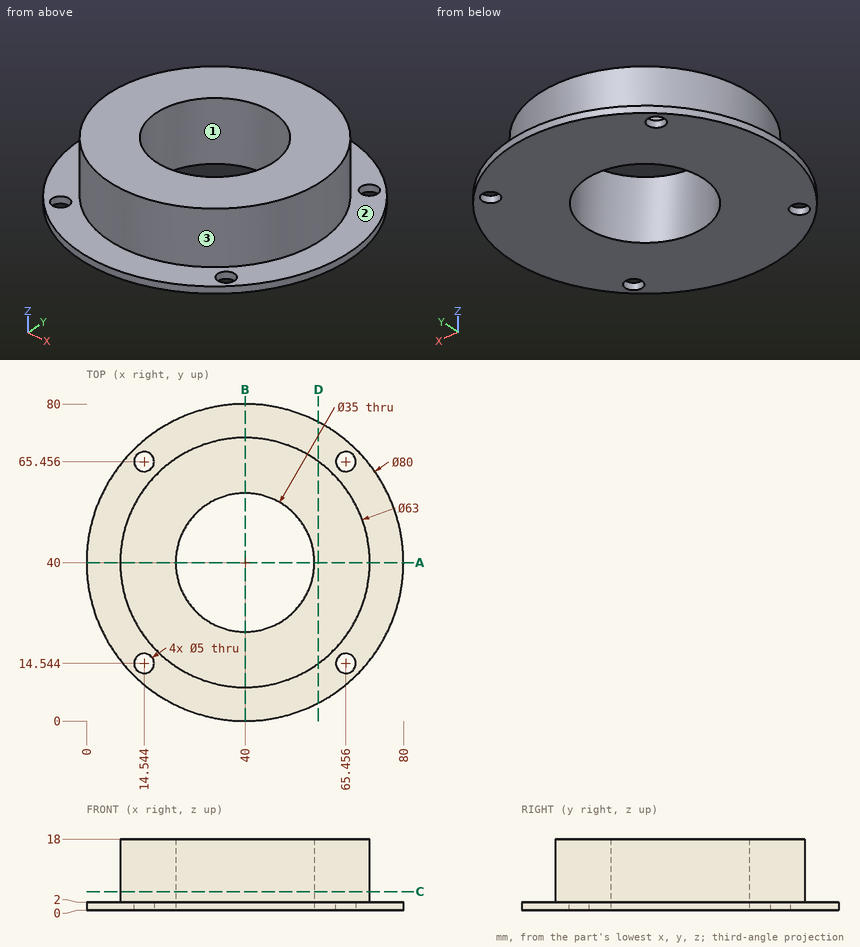
The drawing under review shows one solid part. Ordinate dimensions are in mm from its lowest x, y, z. Coordinates: 2 decimals unless noted, no trailing zeros. Write each loop counter-clockwise with the first axis right and the second up, starting at its lowest first coordinate (ties: lowest second). Pieces come first, ordered by that corner, then holes. Notation, with made-up numbers: (-9, 61) - (7, 61) arc R17 cw to (7, 93) - close; hole circle Ø9 at (34, 47). An arc over 180 degrees is marked (long way). Answer in a Markdown table with one row per item. Add a question column.
Q1. We need section A-A, the plane y = 40. State the section outline as (x, z) points, and give its area (3 significant figures).
Q2. For probe 1 along X at (y, z) = (39.5, 8); probe 2 along Y at (x, z) = (34, 6.75), list the stretches that pass through material, from the lowest coordinate up.
Q3. For P1, Ø3, axis at y = 24.5, z = 5, coming from the -X side; P2, Ø3, axis at y = 66.5, z = 3, coming from the +X side (1 decimal); P3, Ø1, axis at y = 19, z = 7, coming from the +X side, all flat-tipped, find the tip position at first contact; note any pin that passes through.
Q4. We need section D-D, the plane x = 58.5. State the section outline as (y, z) points (1 decimal).
Q5. We need section C-C, the plane z = 4.75. State the section outline as (x, y) points.
Q6. Draft analysis for pull direction Y (two halves, no side actions). For the marked faces 1, 2 and 3, state which applies: +Y half, -Y half, draft (parallel to the pull), parting line (faces both ways), or undercut.
Answer list:
| question | item | result |
|---|---|---|
| 1 | outline | (0, 0) - (22.5, 0) - (22.5, 18) - (8.5, 18) - (8.5, 2) - (0, 2) - close; (57.5, 0) - (80, 0) - (80, 2) - (71.5, 2) - (71.5, 18) - (57.5, 18) - close |
| 1 | area | 538 mm2 |
| 2 | probe 1 | x = 8.5 to 22.51, 57.49 to 71.5 |
| 2 | probe 2 | y = 9.08 to 23.56, 56.44 to 70.92 |
| 3 | P1 | stops at x = 11.78 |
| 3 | P2 | stops at x = 70.9 |
| 3 | P3 | stops at x = 63.92 |
| 4 | outline | (4.5, 0) - (75.5, 0) - (75.5, 2) - (65.5, 2) - (65.5, 18) - (14.5, 18) - (14.5, 2) - (4.5, 2) - close |
| 5 | outline | circle Ø63 at (40, 40); hole circle Ø35 at (40, 40) |
| 6 | face 1 | undercut |
| 6 | face 2 | draft |
| 6 | face 3 | parting line |
